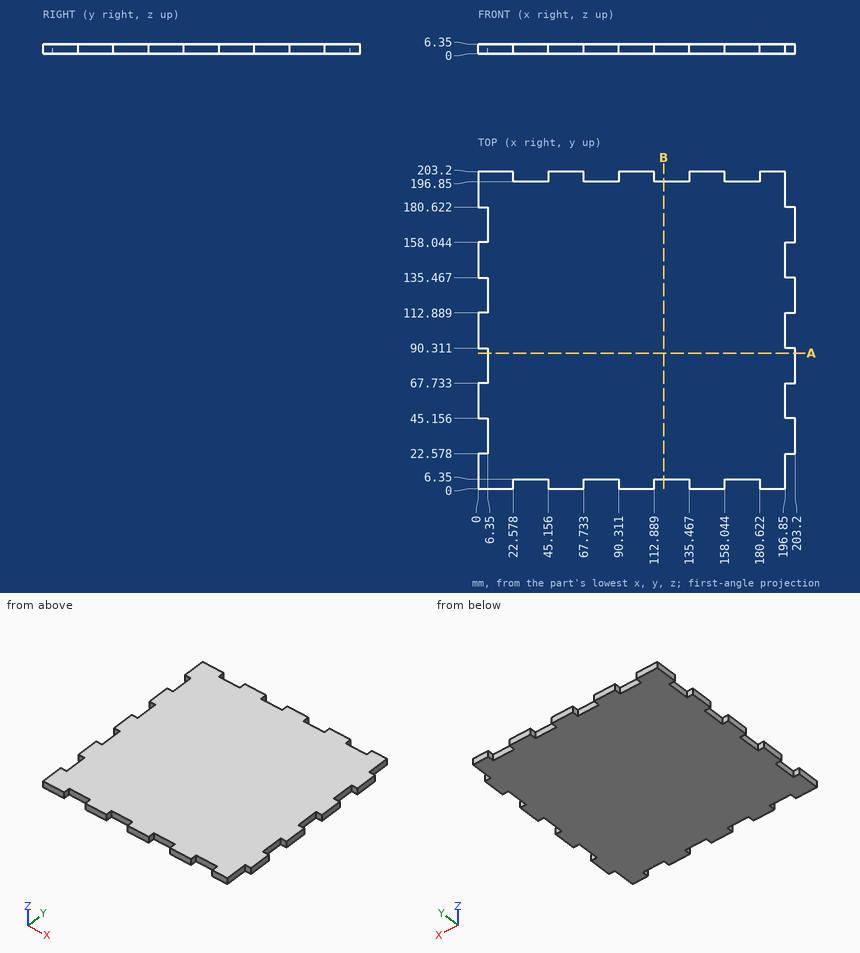
Source: three-view drawing plus pictorial views. Frame: mm from the lowest corner of the part. Coordinates: 2 decimals unless noted, no trailing zeros. Order: outer loops, then holes, each group sorted by start corner. A loop starts at its lowest first (then second) coordinate and runs counter-clockwise, first axis right, second up. Notation, with made-up numbers: (13, 77) -> (57, 77) arc R18 cw to (57, 88) -> close; hole circle Ø9 at (35.5, 10). An arc over 180 degrees is marked (long way). Write item = value, one per line.
(1) Cut plane B-B on x = 119. Return loops of the section in (y, z), plus the area to 3 significant figures.
Solved:
outline = (6.35, 0) -> (196.85, 0) -> (196.85, 6.35) -> (6.35, 6.35) -> close
area = 1,210 mm²
(2) Cut plane A-A on y = 87. Return loops of the section in (x, z).
Solved:
outline = (6.35, 0) -> (203.2, 0) -> (203.2, 6.35) -> (6.35, 6.35) -> close
(3) Line query: line 1 (Y direction, x = 172, z = 1.5); line 2 (X direction, y = 177, z = 4); line 3 (X direction, y = 11.5, z = 2.25). Output: solid intervals per line, ascending.
Solved:
line_1 = 6.35 to 196.85
line_2 = 6.35 to 203.2
line_3 = 0 to 196.85
(4) Pin query (flat end, axial travel): pin 1 Ø3 at (x, z) = (201, 3.5) entering from +Y; pin 2 Ø1.9 at (y, z) = (3, 4) entering from -X; pin 3 Ø1.9 at (x, z) = (36.5, 2) entering from -Y; pin 4 Ø3 at (y, z) = (125.5, 4) entering from -X. Return the tip coordinate at first contact, or that it passes through.
Solved:
pin_1 = 180.62
pin_2 = 0
pin_3 = 6.35
pin_4 = 6.35
